Check sheet for the drawn part. Datum: minimum x, y, z corner. Units: mm. A direction names the side the tool comes from. Coordinates: 2 decimals unless noted, no trailing zeros. Loops run counter-clockwise (first coordinate to the right, second up) from the corner with the lowest first, then second, coordinate; pieces in that order, holes last. Notation, with made-up numbers: (6, -25.75) -> (31, -25.75) arc R18 cw to (31, -13.75) -> close; hole circle Ø6 at (29.25, -12.5). An arc over 180 degrees is marked (long way). Use CSV: the item, a comma, the result in double quotes. Start each with the question number.
1. Sectioned sample at D-D, the plane z = 2. Record the cut outline in (x, y).
2. Set-up check for the marked faces 4 and 5: record each of +Z, -Z, +X, -X, +Y, -Y from which the full face is reachable in a straight line by a thin tool's end or side.
3. Gauge pin test, flat ends, axial feed: pin 1 (6 mm diameter, centred on y = 17.5, z = 1, fed in from +X); pin 2 (6.5 mm diameter, centred on x = 12.5, y = 12.5, fed in from -Z); pin 3 (6 mm diameter, centred on y = 5.5, z = 8.5, fed in from -X). Record the tip position at first contact, or that the pin passes through.
4. Release check for a two-part mould opening along Y. For the marked faces 1, 2 and 3 record: pulls with the +Y half, pulls with the -Y half, needs draft (parallel to the pull), parting line crosses it, or undercut.
5. Sectioned sample at B-B, the plane x = 12.5. Record the cut outline in (y, z).
6. Sectioned sample at A-A, the plane x = 5.25. Record the cut outline in (y, z).
7. Thickness scan on L1, parallel to X at y = 12.25, z = 0.75; L2, parallel to X at y = 12.75, z = 10.25; L3, parallel to Y at x = 10.5, z = 6 (1 decimal). Record the ranges inside material, lowest first.
8. Sectioned sample at C-C, the plane z = 11.25. Record the cut outline in (x, y).
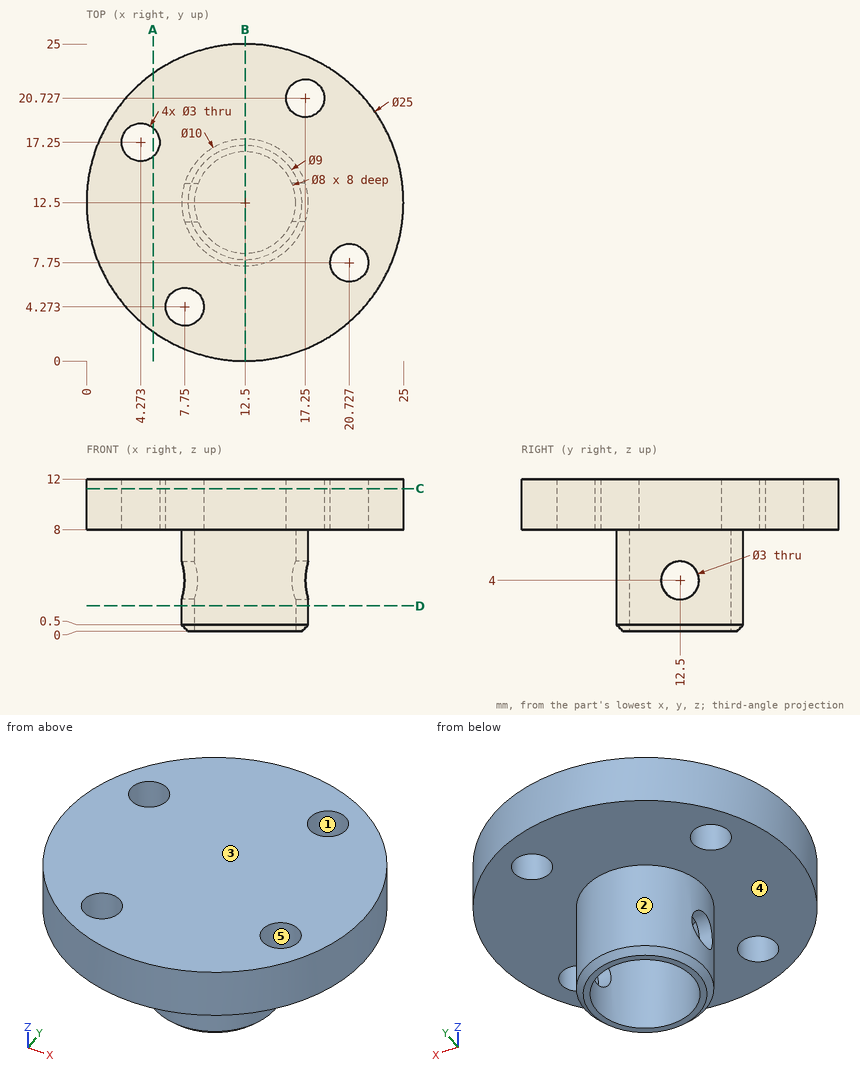
Completed:
1,outline,"circle Ø10 at (12.5, 12.5); hole circle Ø8 at (12.5, 12.5)"
2,face 4,"-Z"
2,face 5,"+Z, -Z"
3,pin 1,"x = 17.08"
3,pin 2,"z = 8"
3,pin 3,"x = 0.66"
4,face 1,"undercut"
4,face 2,"parting line crosses it"
4,face 3,"needs draft"
5,outline,"(0, 8) -> (7.5, 8) -> (7.5, 0.5) -> (8, 0) -> (8.5, 0) -> (8.5, 8) -> (16.5, 8) -> (16.5, 0) -> (17, 0) -> (17.5, 0.5) -> (17.5, 8) -> (25, 8) -> (25, 12) -> (0, 12) -> close"
6,outline,"(2.32, 8) -> (16.11, 8) -> (16.11, 12) -> (2.32, 12) -> close; (18.39, 8) -> (22.68, 8) -> (22.68, 12) -> (18.39, 12) -> close"
7,L1,"7.51 to 8.51, 16.49 to 17.49"
7,L2,"0 to 25"
7,L3,"7.9 to 9, 16 to 17.1"
8,outline,"circle Ø25 at (12.5, 12.5); hole circle Ø3 at (4.27, 17.25); hole circle Ø3 at (7.75, 4.27); hole circle Ø3 at (17.25, 20.73); hole circle Ø3 at (20.73, 7.75)"
